Source: CAD feature listing. Evaluate the final solid. Frame: model axes, mm. A direction names the side the tool comes from. Give positions to 0.01 mm unless a question says otherwise; leave off trailing zeros. Write each loop counter-clockwise with the first axis right and the second up, starting at its lowest first coordinate (ties: lowest second). Pieces come first, ordered by that corner, then holes.
```python
from build123d import *

# Parameters (mm, degrees)
SKETCH_1_R          = 1.65
EXTRUDE_1_DEPTH     = 4
EXTRUDE_START       = 4
SKETCH_2_W          = 40
SKETCH_2_H          = 4
EXTRUDE_2_DEPTH     = 98.5
EXTRUDE_START_2     = 49
SKETCH_4_W          = 40
SKETCH_4_H          = 4
EXTRUDE_3_DEPTH     = 60
FILLET_1_R          = 20
CUT_EXTRUDE_2_DEPTH = 109.310895112
CUT_EXTRUDE_START   = -90.5
SKETCH_8_R          = 5.1
CUT_EXTRUDE_3_DEPTH = 10


with BuildPart() as part:
    # 草图1 → 凸台-拉伸1 (new body)
    with BuildSketch(Plane.XY):
        Polygon((-20, 0), (-20, -15), (20, -15), (20, 3.147792708), (20, 45), (-20, 45), align=None)
        with Locations((-10, 0)):
            Circle(SKETCH_1_R, mode=Mode.SUBTRACT)
        with Locations((0, 10)):
            Circle(SKETCH_1_R, mode=Mode.SUBTRACT)
        with Locations((0, -10)):
            Circle(SKETCH_1_R, mode=Mode.SUBTRACT)
        with Locations((10, 0)):
            Circle(SKETCH_1_R, mode=Mode.SUBTRACT)
    extrude(amount=EXTRUDE_1_DEPTH)

    # 草图2 → 凸台-拉伸2 (add)
    with BuildSketch(Plane.XY.offset(EXTRUDE_START)):
        with Locations((0, 47)):
            Rectangle(SKETCH_2_W, SKETCH_2_H)
    extrude(amount=-EXTRUDE_2_DEPTH)

    # 草图4 → 凸台-拉伸3 (add)
    with BuildSketch(Plane(origin=(0, 0, 0), x_dir=(1, 0, 0), z_dir=(0, 1, 0)).offset(EXTRUDE_START_2)):
        with Locations((0, 92.5)):
            Rectangle(SKETCH_4_W, SKETCH_4_H)
    extrude(amount=-EXTRUDE_3_DEPTH)

    # 圆角1
    fillet_1_edges = [part.edges().sort_by_distance(p)[0] for p in [
        (-20, -11, -92.5),
        (20, -11, -92.5),
        (20, -15, 2),
        (-20, -15, 2),
    ]]
    fillet(fillet_1_edges, radius=FILLET_1_R - 0.0001)  # a hair under: the kernel refuses the full size

    # 草图6 → 切除-拉伸2 (cut, through all)
    with BuildSketch(Plane(origin=(0, 0, 0), x_dir=(1, 0, 0), z_dir=(0, 1, 0))):
        with BuildLine():
            Line((-8.65, 16), (-8.65, 76))
            ThreePointArc((-8.65, 76), (-7, 77.65), (-5.35, 76))
            Line((-5.35, 76), (-5.35, 16))
            ThreePointArc((-5.35, 16), (-7, 14.35), (-8.65, 16))
        make_face()
        with BuildLine():
            Line((1.634526819, 76), (1.634526819, 16))
            ThreePointArc((1.634526819, 16), (0, 14.365473181), (-1.634526819, 16))
            Line((-1.634526819, 16), (-1.634526819, 76))
            ThreePointArc((-1.634526819, 76), (0, 77.634526819), (1.634526819, 76))
        make_face()
        with BuildLine():
            Line((8.598187679, 76), (8.598187679, 16))
            ThreePointArc((8.598187679, 16), (7, 14.401812321), (5.401812321, 16))
            Line((5.401812321, 16), (5.401812321, 76))
            ThreePointArc((5.401812321, 76), (7, 77.598187679), (8.598187679, 76))
        make_face()
    extrude(amount=CUT_EXTRUDE_2_DEPTH, mode=Mode.SUBTRACT)

    # 草图8 → 切除-拉伸3 (cut)
    with BuildSketch(Plane.XY.offset(CUT_EXTRUDE_START)):
        Circle(SKETCH_8_R)
    extrude(amount=-CUT_EXTRUDE_3_DEPTH, mode=Mode.SUBTRACT)


solid = part.part
```
1. Access query for faces 1 (the flat face through (20, 46, -45)), 2 (the cylindrical face through (0.036, 46.972, -14.366)), 3 (the cylindrical face through (2.4, -4.5, -92.5)), 4 (the cylindrical face through (-0.4, 8.4, 2)), 5 (the cylindrical face through (-14.297, -4.986, -92.528)). Directions: +Z, -Z, +X, -X, +Y, -Y. A direction counts if a zero-diameter tool reaches every point of the face in a straight line with its end or side. Return the directions, or none.
2. Cut plane D-D, the plane z = -5. Return the cut outline in (x, y).
3. Cut plane B-B, the plane y = 15. Return the cut outline in (x, z), then the cut area to 3 significant figures.
4. Cut plane C-C, the plane x = -7. Return the cut outline in (y, z), then the cut area to 3 significant figures.
5. Mould query, pull axis Z, two halves, no side actions, for faces 6 (the flat face through (-20, 46, -45)), 7 (the flat face through (0, 15, 0)), 8 (the flat face through (-5, 45, -45)), 9 (the flat face through (0, 19, -94.5)). Classes: +Z half, -Z half, draft (parallel to the pull), parting line (faces both ways), or undercut.
6. Cut plane A-A, the plane z = -68. Return the cut outline in (x, y).
7. Contact query for flat-ended pins moving along their axis: P1, Ø6, axis at x = 0, y = 0, coming from the -Z side; P2, Ø8, axis at x = -13.5, z = -43, coming from the -Y side; P3, Ø2.5, axis at x = -10, y = 0, coming from the +Z side. Output: stop coordinate, or through.
8. Line query: L1, parallel to Z at x = 16.5, y = 1.5; L2, parallel to Y at x = 0, z = -93; L3, parallel to Y at x = 13, z = -74.5. Output: solid intervals per line, ascending.
Response values:
1. face 1: +Z, -Z, +X, +Y, -Y
1. face 2: +Y, -Y
1. face 3: -Z
1. face 4: +Z
1. face 5: -Z, -X, -Y
2. outline: (-20, 45) - (20, 45) - (20, 49) - (-20, 49) - close
3. outline: (-20, -94.5) - (20, -94.5) - (20, -90.5) - (-20, -90.5) - close; (-20, 0) - (20, 0) - (20, 4) - (-20, 4) - close
3. area: 320 mm2
4. outline: (-13.74, 0) - (45, 0) - (45, -14.35) - (49, -14.35) - (49, 4) - (-13.74, 4) - close; (-9.74, -94.5) - (49, -94.5) - (49, -77.65) - (45, -77.65) - (45, -90.5) - (-9.74, -90.5) - close
4. area: 595 mm2
5. face 6: draft
5. face 7: undercut
5. face 8: undercut
5. face 9: -Z half
6. outline: (-20, 45) - (-8.65, 45) - (-8.65, 49) - (-20, 49) - close; (-5.35, 45) - (-1.63, 45) - (-1.63, 49) - (-5.35, 49) - close; (1.63, 45) - (5.4, 45) - (5.4, 49) - (1.63, 49) - close; (8.6, 45) - (20, 45) - (20, 49) - (8.6, 49) - close
7. P1: stops at z = 0
7. P2: stops at y = 45
7. P3: stops at z = -90.5
8. L1: z = -94.5 to -90.5, 0 to 4
8. L2: y = -11 to -5.1, 5.1 to 49
8. L3: y = 45 to 49
